The model under review builds one solid part; all positions refer to its coordinate system, in mm. Face numbers are marked on the shaded views. A direction names the side the tool comes from. Round coordinates to 2 decimals unless told otherwise and drop trailing zeros. Order: outer loops, then holes, each group sorted by start corner. A loop starts at its lowest first (then second) coordinate and runs counter-clockwise, first axis right, second up.
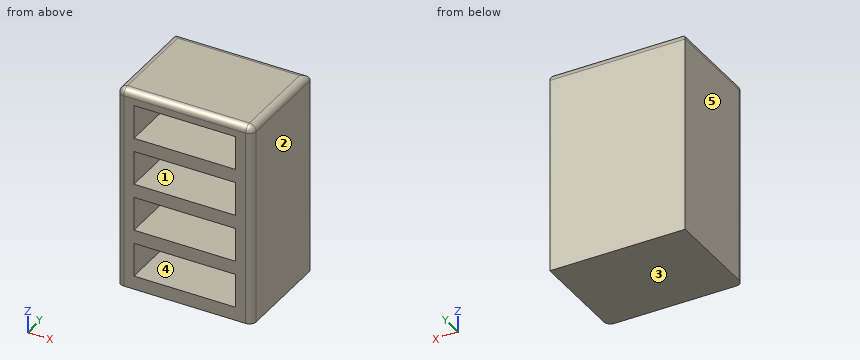
from build123d import *

# Parameters (mm, degrees)
F0_W     = 101.6
F0_H     = 76.2
F1_DEPTH = 152.4
F2_W     = 76.2
F2_H     = 25.4
F3_DEPTH = 50.8
F4_R     = 5.08


with BuildPart() as f1:
    # F0 (on Top) → F1 (new body)
    with BuildSketch(Plane.XY):
        with Locations((50.8, 38.1)):
            Rectangle(F0_W, F0_H)
    extrude(amount=F1_DEPTH)

    # F2 (on face) → F3 (cut)
    with BuildSketch(Plane.XZ):
        with Locations((50.8, 129.54)):
            Rectangle(F2_W, F2_H)
        with Locations((50.8, 93.98)):
            Rectangle(F2_W, F2_H)
        with Locations((50.8, 58.42)):
            Rectangle(F2_W, F2_H)
        with Locations((50.8, 22.86)):
            Rectangle(F2_W, F2_H)
    extrude(amount=-F3_DEPTH, mode=Mode.SUBTRACT)

    # F4
    f4_edges = [f1.edges().sort_by_distance(p)[0] for p in [
        (101.6, 38.1, 152.4),
        (0, 38.1, 152.4),
        (50.8, 0, 152.4),
        (50.8, 76.2, 152.4),
        (101.6, 0, 76.2),
        (0, 0, 76.2),
    ]]
    fillet(f4_edges, radius=F4_R)


solid = f1.part
(1) We need section A-A (y = 29.5). Give the boundary of the cut face in (x, z), and give its area (3 significant figures).
(2) We need section C-C (x = 23.5). Give the boundary of the cut face in (y, z), and give its area (3 significant figures).
(3) The part is to be moulded in two halves that separate along Z. For the marked faces 1, 2 and 3, say which applies: pulls with the +Z half, pulls with the -Z half, needs draft (parallel to the pull), parting line crosses it, or undercut.
(4) To check wall thickness, follow L1, parallel to Z at x = 60.5, y = 23; L2, parallel to X at y = 18.5, z = 84.5; L3, parallel to Y at x = 86, z = 59.5. State the ranges of each line that lie inside material, in increasing order.
(5) Tool access review of the marked faces 4 and 5: name each direction out of +Z, -Z, +X, -X, +Y, -Y from which nothing blocks a thin tool from reaching the whole face with its end or side.
(6) Clearance check with a flat-ended pin moving along its axis: P1, Ø12, axis at x = 35, z = 90, coming from the -Y side. State where the tip first meets the part, or that it passes through.
(7) We need section B-B (z = 15). Give the boundary of the cut face in (x, y), and give its area (3 significant figures).
Verdict:
1. outline: (0, 0) - (101.6, 0) - (101.6, 147.32) arc R5.08 ccw to (96.52, 152.4) - (5.08, 152.4) arc R5.08 ccw to (0, 147.32) - close; hole (12.7, 10.16) - (88.9, 10.16) - (88.9, 35.56) - (12.7, 35.56) - close; hole (12.7, 45.72) - (88.9, 45.72) - (88.9, 71.12) - (12.7, 71.12) - close; hole (12.7, 81.28) - (88.9, 81.28) - (88.9, 106.68) - (12.7, 106.68) - close; hole (12.7, 116.84) - (88.9, 116.84) - (88.9, 142.24) - (12.7, 142.24) - close
1. area: 7,730 mm2
2. outline: (0, 0) - (76.2, 0) - (76.2, 147.32) arc R5.08 ccw to (71.12, 152.4) - (5.08, 152.4) arc R5.08 ccw to (0, 147.32) - (0, 142.24) - (50.8, 142.24) - (50.8, 116.84) - (0, 116.84) - (0, 106.68) - (50.8, 106.68) - (50.8, 81.28) - (0, 81.28) - (0, 71.12) - (50.8, 71.12) - (50.8, 45.72) - (0, 45.72) - (0, 35.56) - (50.8, 35.56) - (50.8, 10.16) - (0, 10.16) - close
2. area: 6,440 mm2
3. face 1: undercut
3. face 2: needs draft
3. face 3: pulls with the -Z half
4. L1: z = 0 to 10.16, 35.56 to 45.72, 71.12 to 81.28, 106.68 to 116.84, 142.24 to 152.4
4. L2: x = 0 to 12.7, 88.9 to 101.6
4. L3: y = 50.8 to 76.2
5. face 4: -Y
5. face 5: +Z, -Z, -X, +Y, -Y
6. P1: stops at y = 50.8
7. outline: (0, 5.08) arc R5.08 ccw to (5.08, 0) - (12.7, 0) - (12.7, 50.8) - (88.9, 50.8) - (88.9, 0) - (96.52, 0) arc R5.08 ccw to (101.6, 5.08) - (101.6, 76.2) - (0, 76.2) - close
7. area: 3,860 mm2
